The drawing under review shows one solid part. Ordinate dimensions are in mm from its lowest x, y, z. Give positions to 0.01 mm unless a question says otherwise; leave off trailing zeros. Order: outer loops, then holes, each group sorted by start corner. A loop starts at its lowest first (then second) coordinate and runs counter-clockwise, first axis right, second up. Notation, with made-up numbers: (14.5, 83) - (73.5, 83) arc R27 ccw to (73.5, 113) - close; hole circle Ø1 at (77, 88.25). An arc over 180 degrees is marked (long way). Use CSV: the item, a comma, the result in double quotes. Start each with the question number.
1. For pin 1 (9.5 mm diameter, centred on x = 209.75, y = 39.9, fed in from -Z); pin 2 (3 mm diameter, centred on y = 253, z = 2, fed in from +X) (1 decimal); pin 3 (1.5 mm diameter, centred on y = 218.5, z = 6, fed in from -X) (1 decimal); pin 4 (6 mm diameter, centred on x = 221.5, z = 3.5, fed in from -Y), all flat-tipped, find the tip position at first contact; note any pin that passes through.
2. Take a section at D-D, the plane y = 112. State the section outline as (x, z) points (1 decimal), then the cut area to 3 significant figures.
3. Take a section at A-A, the plane x = 160. State the section outline as (y, z) points, then the cut area to 3 significant figures.
4. Take a section at C-C, the plane z = 3. Count the separate pieces of the cut face and the enclosed holes in it, then the cut area to 3 significant figures.
5. To check wall thickness, follow line 1 (Y direction, x = 160, z = 6.75); line 2 (Y direction, x = 117, z = 6.25); line 3 (X direction, y = 183, z = 9). State the ranges of each line that lie inside material, in increasing order. Write a range as [from, to].
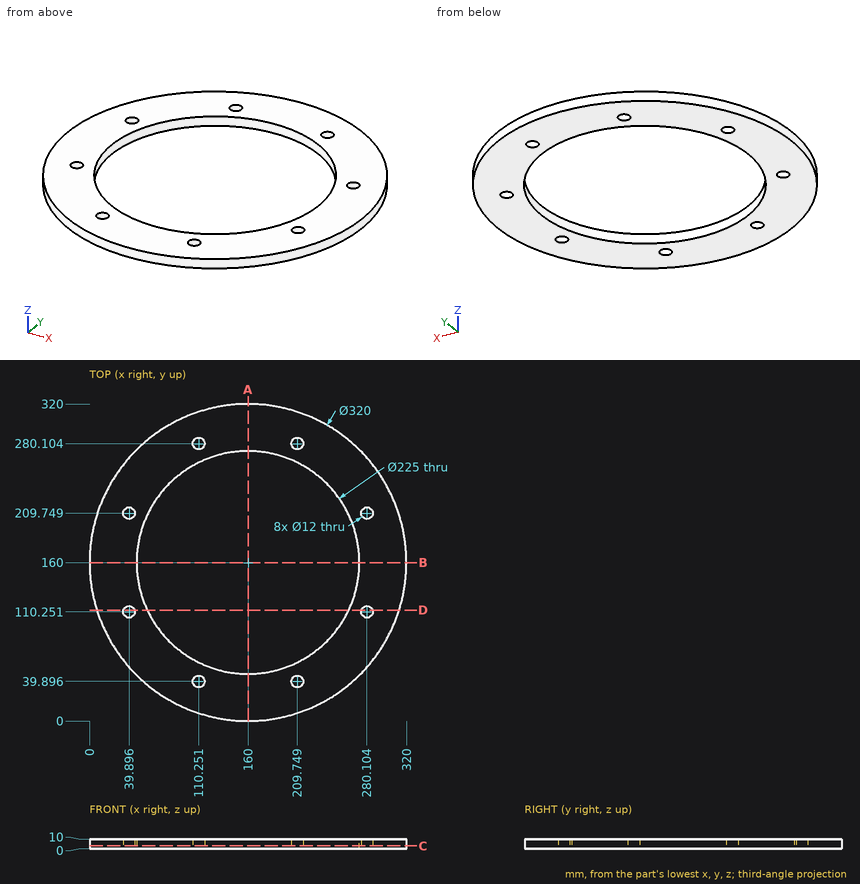
Determined:
1,pin 1,"passes through"
1,pin 2,"stops at x = 291.3"
1,pin 3,"stops at x = 10.8"
1,pin 4,"stops at y = 11.08"
2,outline,"(7.4, 0) - (34.2, 0) - (34.2, 10) - (7.4, 10) - close; (45.6, 0) - (58.3, 0) - (58.3, 10) - (45.6, 10) - close; (261.7, 0) - (274.4, 0) - (274.4, 10) - (261.7, 10) - close; (285.8, 0) - (312.6, 0) - (312.6, 10) - (285.8, 10) - close"
2,area,"788 mm²"
3,outline,"(0, 0) - (47.5, 0) - (47.5, 10) - (0, 10) - close; (272.5, 0) - (320, 0) - (320, 10) - (272.5, 10) - close"
3,area,"950 mm²"
4,separate pieces,"1"
4,enclosed holes,"9"
4,area,"39,800 mm²"
5,line 1,"y = [0, 47.5], [272.5, 320]"
5,line 2,"y = [5.89, 56.04], [263.96, 314.11]"
5,line 3,"x = [1.66, 49.88], [270.12, 318.34]"
